Design review of the part built by this model. Coordinates are the model's own, in mm. A direction names the side the tool comes from. Round coordinates to 2 decimals unless told otherwise and drop trailing zeros. Order: outer loops, then holes, each group sorted by start corner. A loop starts at its lowest first (then second) coordinate and runs counter-clockwise, first axis right, second up.
from build123d import *

# Parameters (mm, degrees)
F1_DEPTH = 5.842
F2_R     = 3.175
F3_DEPTH = 5.842


# Not quite as in the source:
# - a feature names something its author has since deleted; it is built from what else it names


with BuildPart() as f1:
    # F0 (on Top) → F1 (new body)
    with BuildSketch(Plane.XY):
        with BuildLine():
            Line((-37.108954253, 15.875), (-43.458954253, 15.875))
            Line((-43.458954253, 15.875), (-75.208954253, 15.875))
            ThreePointArc((-75.208954253, 15.875), (-79.6990823135, 14.0151280605), (-81.558954253, 9.525))
            Line((-81.558954253, 9.525), (-81.558954253, -28.575))
            ThreePointArc((-81.558954253, -28.575), (-79.6990823135, -33.0651280605), (-75.208954253, -34.925))
            Line((-75.208954253, -34.925), (-72.710875161, -34.925))
            Line((-72.710875161, -34.925), (-56.7378558105, -50.8045013442))
            Line((-56.7378558105, -50.8045013442), (10.8431089825, -117.9897966054))
            ThreePointArc((10.8431089825, -117.9897966054), (21.0344920397, -66.1580316621), (64.9777384297, -95.4733389685))
            ThreePointArc((64.9777384297, -95.4733389685), (62.5609135869, -107.6235379461), (55.6783787323, -117.9239792712))
            Line((55.6783787323, -117.9239792712), (110.9403548131, -62.6620031905))
            Line((110.9403548131, -62.6620031905), (138.6796593377, -34.9226986659))
            Line((138.6796593377, -34.9226986659), (140.691045747, -34.9226986659))
            ThreePointArc((140.691045747, -34.9226986659), (145.1811738076, -33.0628267264), (147.041045747, -28.5726986659))
            Line((147.041045747, -28.5726986659), (147.041045747, 9.525))
            ThreePointArc((147.041045747, 9.525), (145.1811738076, 14.0151280605), (140.691045747, 15.875))
            Line((140.691045747, 15.875), (108.941045747, 15.875))
            Line((108.941045747, 15.875), (102.591045747, 15.875))
            ThreePointArc((102.591045747, 15.875), (98.1009176865, 14.0151280605), (96.241045747, 9.525))
            Line((96.241045747, 9.525), (96.241045747, 0))
            Line((96.241045747, 0), (90.399045747, 0))
            Line((90.399045747, 0), (90.399045747, -19.05))
            Line((90.399045747, -19.05), (97.2144311123, -19.05))
            Line((97.2144311123, -19.05), (97.2144311123, -34.925))
            Line((97.2144311123, -34.925), (88.2341749912, -43.9052561211))
            Line((88.2341749912, -43.9052561211), (-21.7786981319, -43.9052561211))
            Line((-21.7786981319, -43.9052561211), (-30.758954253, -34.925))
            Line((-30.758954253, -34.925), (-30.758954253, -19.05))
            Line((-30.758954253, -19.05), (-24.916954253, -19.05))
            Line((-24.916954253, -19.05), (-24.916954253, 0))
            Line((-24.916954253, 0), (-30.758954253, 0))
            Line((-30.758954253, 0), (-30.758954253, 9.525))
            ThreePointArc((-30.758954253, 9.525), (-32.6188261924, 14.0151280605), (-37.108954253, 15.875))
        make_face()
        with BuildLine():
            ThreePointArc((64.9777384297, -95.4733389685), (21.0344920397, -66.1580316621), (10.8431089825, -117.9897966054))
            ThreePointArc((10.8431089825, -117.9897966054), (33.2743467834, -127.2233047585), (55.6783787323, -117.9239792712))
            ThreePointArc((55.6783787323, -117.9239792712), (62.5609135869, -107.6235379461), (64.9777384297, -95.4733389685))
        make_face()
    extrude(amount=F1_DEPTH)

    # F2 (on face) → F3 (cut, through all)
    with BuildSketch(Plane.XY.offset(5.842)):
        with Locations((33.2277384297, -95.4733389685)):
            Circle(F2_R)
    extrude(amount=-F3_DEPTH, mode=Mode.SUBTRACT)


solid = f1.part
1) Clearance check with flat-ended pins moving along their axes: P1, Ø12, axis at x = 65, y = -98.5, coming from the -Z side; P2, Ø0.6, axis at x = 140, z = 4, coming from the -Y side; P3, Ø3, axis at x = 93, z = 2.5, coming from the +Y side; P4, Ø3, axis at y = -80.5, z = 1.5, coming from the +X side. State where each tip first meets the part, or that it passes through.
Results:
P1: stops at z = 0
P2: stops at y = -34.92
P3: stops at y = 0
P4: stops at x = 94.6
2) To check wall thickness, follow line 1 along X through (y, z) = (8.5, 3.2); line 2 along X through (y, z) = (-1.5, 0.8); line 3 along Y through (x, z) = (-12, 4.35). State the ranges of each line that lie inside material, in increasing order.
Results:
line 1: x = -81.56 to -30.76, 96.24 to 147.04
line 2: x = -81.56 to -24.92, 90.4 to 147.04
line 3: y = -95.28 to -43.91
3) For faces 1 (the face through (-26.206, -39.478, 2.88)), 2 (the face through (32.93, -127.22, 2.88)), 3 (the face through (34, -43.905, 3)), list the 3-axis set-ups (+Z, -Z, +X, -X, +Y, -Y) from which the entire face can be reached by the end or side of a thin tool; tool diameter is ignored.
Results:
face 1: +Z, -Z
face 2: +Z, -Z, -Y
face 3: +Z, -Z, +Y
4) Take a section at C-C on y = -80. Give the boundary of the cut face in (x, z).
Results:
outline: (-27.37, 0) - (93.6, 0) - (93.6, 5.84) - (-27.37, 5.84) - close
5) Take a section at D-D on x = -59. Give the boundary of the cut face in (y, z) (3 decimals), plus the area to 3 significant figures.
Results:
outline: (-48.556, 0) - (15.875, 0) - (15.875, 5.842) - (-48.556, 5.842) - close
area: 376 mm2
6) The part is to be moulded in two halves that separate along Y. For faces 4 (the face through (31, -55, 0)), 5 (the face through (145.23, 13.965, 2.88)), 6 (the face through (92.79, -39.35, 2.88)), say which applies: released by +Y, released by -Y, zero draft, split by the parting line, or undercut.
Results:
face 4: zero draft
face 5: released by +Y
face 6: undercut
7) Take a section at A-A on y = 3.5. Give the boundary of the cut face in (x, z), plus the area to 3 significant figures.
Results:
outline: (-81.56, 0) - (-30.76, 0) - (-30.76, 5.84) - (-81.56, 5.84) - close; (96.24, 0) - (147.04, 0) - (147.04, 5.84) - (96.24, 5.84) - close
area: 594 mm2
